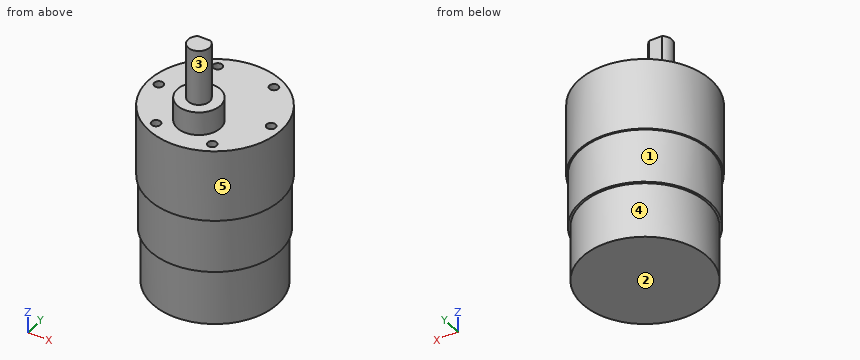
```python
from build123d import *

# Parameters (mm, degrees)
SKETCH1_R                       = 17.4
BOSS_EXTRUDE1_DEPTH             = 15.4
SKETCH2_R                       = 18
BOSS_EXTRUDE2_DEPTH             = 15
SKETCH3_R                       = 18.4
BOSS_EXTRUDE3_DEPTH             = 20
SKETCH4_R                       = 6
BOSS_EXTRUDE4_DEPTH             = 6.5
SKETCH5_R                       = 3
BOSS_EXTRUDE5_DEPTH             = 15.5
CUT_EXTRUDE1_DEPTH              = 13
TAP_DRILL_FOR_M3X0_5_TAP1_D     = 2.5
TAP_DRILL_FOR_M3X0_5_TAP1_DEPTH = 10.76


with BuildPart() as part:
    # Sketch1 → Boss-Extrude1 (new body)
    with BuildSketch(Plane.XY):
        Circle(SKETCH1_R)
    extrude(amount=BOSS_EXTRUDE1_DEPTH)

    # Sketch2 → Boss-Extrude2 (add)
    with BuildSketch(Plane.XY.offset(15.4)):
        Circle(SKETCH2_R)
    extrude(amount=BOSS_EXTRUDE2_DEPTH)

    # Sketch3 → Boss-Extrude3 (add)
    with BuildSketch(Plane.XY.offset(30.4)):
        Circle(SKETCH3_R)
    extrude(amount=BOSS_EXTRUDE3_DEPTH)

    # Sketch4 → Boss-Extrude4 (add)
    with BuildSketch(Plane.XY.offset(50.4)):
        with Locations((0, -7)):
            Circle(SKETCH4_R)
    extrude(amount=BOSS_EXTRUDE4_DEPTH)

    # Sketch5 → Boss-Extrude5 (add)
    with BuildSketch(Plane.XY.offset(56.9)):
        with Locations((0, -7)):
            Circle(SKETCH5_R)
    extrude(amount=BOSS_EXTRUDE5_DEPTH)

    # Sketch6 → Cut-Extrude1 (cut)
    with BuildSketch(Plane.XY.offset(72.4)):
        with BuildLine():
            Line((-1.8, -4.6), (1.8, -4.6))
            ThreePointArc((1.8, -4.6), (0, -4), (-1.8, -4.6))
        make_face()
    extrude(amount=-CUT_EXTRUDE1_DEPTH, mode=Mode.SUBTRACT)

    # Tap Drill for M3x0.5 Tap1
    with Locations(Plane.XY.offset(50.4)):
        with Locations((-15.5, 0), (-7.75, 13.423393759), (7.75, 13.423393759), (15.5, 0), (7.75, -13.423393759), (-7.75, -13.423393759)):
            Hole(TAP_DRILL_FOR_M3X0_5_TAP1_D / 2, depth=TAP_DRILL_FOR_M3X0_5_TAP1_DEPTH)


solid = part.part
```
Input: part model. Units: mm. Frame: model coordinates. Face numbers are marked on the shaded views. A direction names the side the tool comes from. Give positions to 0.01 mm unless a question says otherwise; leave off trailing zeros. Order: outer loops, then holes, each group sorted by start corner. A loop starts at its lowest first (then second) coordinate and runs counter-clockwise, first axis right, second up.
1. Section B-B on y = 4. Return the cut outline in (x, z), and give its area (3 significant figures).
Derived:
outline: (-17.96, 30.4) - (-17.55, 30.4) - (-17.55, 15.4) - (-16.93, 15.4) - (-16.93, 0) - (16.93, 0) - (16.93, 15.4) - (17.55, 15.4) - (17.55, 30.4) - (17.96, 30.4) - (17.96, 50.4) - (-17.96, 50.4) - close
area: 1,770 mm2
2. Mould query, pull axis X, two halves, no side actions, for the marked faces 1 and 2. Classes: released by +X, released by -X, zero draft, split by the parting line, or undercut.
Derived:
face 1: split by the parting line
face 2: zero draft
3. Section C-C on z = 21.5. Return the cut outline in (x, y).
Derived:
outline: circle Ø36 at (0, 0)
4. Section D-D on y = -2. Return the cut outline in (x, z).
Derived:
outline: (-18.29, 30.4) - (-17.89, 30.4) - (-17.89, 15.4) - (-17.28, 15.4) - (-17.28, 0) - (17.28, 0) - (17.28, 15.4) - (17.89, 15.4) - (17.89, 30.4) - (18.29, 30.4) - (18.29, 50.4) - (3.32, 50.4) - (3.32, 56.9) - (-3.32, 56.9) - (-3.32, 50.4) - (-18.29, 50.4) - close
5. Section A-A on x = 7.75. Return the cut outline in (y, z).
Derived:
outline: (-16.69, 30.4) - (-16.25, 30.4) - (-16.25, 15.4) - (-15.58, 15.4) - (-15.58, 0) - (15.58, 0) - (15.58, 15.4) - (16.25, 15.4) - (16.25, 30.4) - (16.69, 30.4) - (16.69, 50.4) - (14.67, 50.4) - (14.67, 39.64) - (12.17, 39.64) - (12.17, 50.4) - (-12.17, 50.4) - (-12.17, 39.64) - (-14.67, 39.64) - (-14.67, 50.4) - (-16.69, 50.4) - close
6. Reachability of the marked faces 3, 4 and 5 from +Z, -Z, +X, -X, +Y, -Y: full face, straight path, thin tool, end or side. Return the list, or none.
Derived:
face 3: +Z
face 4: -Z
face 5: +Z, -Z
7. Pin query (flat end, axial travel): pin 1 (10 mm diameter, centred on y = -8.5, z = 62.5, fed in from -X); pin 2 (1.2 mm diameter, centred on x = -8, y = -13.5, fed in from +Z); pin 3 (3 mm diameter, centred on x = -5.5, z = 48, fed in from +Y). Return the tip coordinate at first contact, or that it passes through.
Derived:
pin 1: stops at x = -3
pin 2: stops at z = 39.64
pin 3: stops at y = 17.96
8. Material intervals for L1, parallel to Y at x = -7, z = 44; L2, parallel to Y at x = -7.75, z = 48.25; L3, parallel to Z at x = 10, y = -3, sorted ascending.
Derived:
L1: y = -17.02 to -14.42, -12.42 to 12.42, 14.42 to 17.02
L2: y = -16.69 to -14.67, -12.17 to 12.17, 14.67 to 16.69
L3: z = 0 to 50.4
